```python
from build123d import *

# Parameters (mm, degrees)
SKETCH_1_R           = 12.5
EXTRUDE_1_DEPTH      = 51
SKETCH_2_R           = 4.999511077
EXTRUDE_2_DEPTH      = 5
EXTRUDE_2_DEPTH_BACK = 5


with BuildPart() as part:
    # Sketch 1 → Extrude 1 (new body)
    with BuildSketch(Plane.XY):
        Circle(SKETCH_1_R)
    extrude(amount=EXTRUDE_1_DEPTH)

    # Sketch 2 → Extrude 2 (add, two sides)
    with BuildSketch(Plane(origin=(0, 0, 0), x_dir=(0, 0, -1), z_dir=(0, 1, 0))) as extrude_2_sk:
        with BuildLine():
            Line((-69.235394105, 10.194154198), (-51, 12.5))
            Line((-51, 12.5), (-51, -12.5))
            Line((-51, -12.5), (-69.235394105, -10.194154198))
            ThreePointArc((-69.235394105, -10.194154198), (-79.429548303, 0), (-69.235394105, 10.194154198))
        make_face()
        with Locations((-69.235394105, 0)):
            Circle(SKETCH_2_R, mode=Mode.SUBTRACT)
    extrude(amount=EXTRUDE_2_DEPTH)
    extrude(extrude_2_sk.sketch, amount=-EXTRUDE_2_DEPTH_BACK)


solid = part.part
```
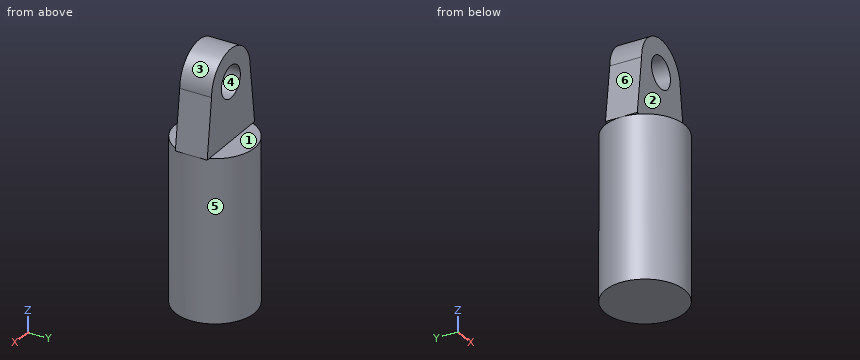
Check sheet for the modelled part. Datum: model origin and axes. Units: mm. Face numbers are marked on the shaded views. A direction names the side the tool comes from. Coordinates: 2 decimals unless noted, no trailing zeros. Order: outer loops, then holes, each group sorted by start corner. A loop starts at its lowest first (then second) coordinate and runs counter-clockwise, first axis right, second up. Notation, with made-up numbers: M 87.5,57 L 96.5,57 A18 cw 96.5,88 Z; hole C -2,46.25 d6. An arc over 180 degrees is marked long. Write each question's results on one line, items separated by ' | '. Start each with the question number.
1. Cross-section at D-D on z = 19. Record the cut outline in (x, y).
2. Cross-section at A-A on x = 0. Record the cut outline in (y, z).
3. Cross-section at C-C on x = 8. Record the cut outline in (y, z).
4. Cross-section at B-B on z = 71.5. Record the cut outline in (x, y), and give its area (3 significant figures).
5. Material ranges on probe 1 along Z at (x, y) = (0, 0.5); probe 2 along Y at (x, z) = (-7, 66); probe 3 along Z at (x, y) = (4.5, 8.75), recorded low to high.
6. Access from +Z, -Z, +X, -X, +Y, -Y to the whole of each face (thin tool, end or side, straight path). Record for the marked faces 1, 2 and 3.
7. Mould release check, pull along X, two halves, no side actions. Record for the marked faces 4, 5 and 6: +X half, -X half, draft (parallel to the pull), parting line (faces both ways), or undercut.
8. Go/stop test with flat-tipped pins: P1, Ø1, axis at x = -5, y = 3.5, coming from the +Z side; P2, Ø8, axis at x = 6, z = 40, coming from the +Y side; P3, Ø4, axis at x = 2, y = 8, coming from the +Z side. Record where each tip stops, or that it passes through.
Checks:
1) outline: C 0,0 d25
2) outline: M -12.5,0 L 12.5,0 L 12.5,51 L 5,51 L 5,64.24 L -5,64.24 L -5,51 L -12.5,51 Z; M -5,74.23 L 5,74.23 L 5,79.43 L -5,79.43 Z
3) outline: M -9.6,0 L 9.6,0 L 9.6,51 L 5,51 L 5,75.55 L -5,75.55 L -5,51 L -9.6,51 Z
4) outline: M -9.94,-5 L -4.46,-5 L -4.46,5 L -9.94,5 Z; M 4.46,-5 L 9.94,-5 L 9.94,5 L 4.46,5 Z | area: 110 mm²
5) probe 1: z = 0 to 64.24, 74.23 to 79.43 | probe 2: y = -5 to 5 | probe 3: z = 0 to 51
6) face 1: +Z, +X, -X, +Y | face 2: +Z, +X, -X, -Y | face 3: +Z, +Y, -Y
7) face 4: undercut | face 5: parting line | face 6: -X half
8) P1: stops at z = 78.38 | P2: stops at y = 12.34 | P3: stops at z = 51
